Here's how the part is built. I have some questions about the finished solid (model axes, mm). A direction names the side the tool comes from. Coordinates: 2 decimals unless noted, no trailing zeros. Order: outer loops, then holes, each group sorted by start corner. A loop starts at its lowest first (then second) coordinate and runs counter-clockwise, first axis right, second up. Notation, with made-up numbers: (64, 69.5) - (95, 69.5) arc R20 cw to (95, 75.5) - close; hole circle Ø8 at (39.25, 10.25). An arc over 180 degrees is marked (long way). Answer in a Markdown table with one row per item. Add a question column.
Item 1: I want a section at A-A (y = -1.75). Please give me the cut outline in (x, z).
Item 2: I want a section at B-B (x = 15). Please give me the cut outline in (y, z), plus the area to 3 significant figures.
Item 3: If I drill on line 1 along Y through (x, z) = (11.5, 16.5); line 2 along Z through (x, y) = (15, -14.05); line 3 along X through (y, z) = (-7.5, 5.75), over which ranges is the centre line in solid material (lowest first)? Write a range as from..to.
Item 4: I want a section at C-C (z = 11.75). Please give me the cut outline in (x, y).
Item 5: I want a section at D-D (z = 18). Please give me the cut outline in (x, y).
Item 6: On a 3-axis mill with a long thin cutter (end or side, diameter ignored), from which of +Z, -Z, +X, -X, +Y, -Y can I reach the whole of each face in a straight line? I mean faces 4 (the flat face through (2.5, -8, 9)), 5 (the flat face through (2, -7, 15)), 6 (the flat face through (22.652, -13.732, 16.332)). Say none if no direction works.
Item 7: Thinking about a two-plate mould opening in Y: for faces 1 (the flat face through (18, -2.5, 7)), 2 (the flat face through (0, -8, 7)), 3 (the flat face through (14, 0, 6)), which applies, +Y half, -Y half, draft (parallel to the pull), parting line (faces both ways), or undercut?
Item 8: Will these pins go through, and if not, where does the flat tip stop? pin 1 Ø2 at (y, z) = (-14.5, 17) entering from -X; pin 2 Ø5 at (x, y) = (4.5, -4.5) entering from -Z; pin 3 Ø2 at (x, y) = (4, -5.5) entering from +Z; pin 4 Ø4 at (x, y) = (29, -12.5) entering from +Z.
```python
from build123d import *

# Parameters (mm, degrees)
F1_DEPTH = 15
F2_W     = 10
F2_H     = 7.5
F2_H_2   = 12.5
F3_DEPTH = 40
F4_R     = 3.75
F5_DEPTH = 29
F6_W     = 2.5
F6_H     = 10
F7_DEPTH = 12.5


with BuildPart() as f1:
    # F0 (on Front) → F1 (new body)
    with BuildSketch(Plane.XZ):
        Polygon((0, 15), (0, 0), (36.2, 0), (28.829492, 12.766094), (16.3, 20), (7.5, 20), (7.5, 15), align=None)
    extrude(amount=F1_DEPTH)

    # F2 (on face) → F3 (cut)
    with BuildSketch(Plane(origin=(0, 0, 0), x_dir=(0, -1, 0), z_dir=(-1, 0, 0))):
        with Locations((7.5, 18.75)):
            Rectangle(F2_W, F2_H)
        with Locations((7.5, 8.75)):
            Rectangle(F2_W, F2_H_2)
    extrude(amount=-F3_DEPTH, mode=Mode.SUBTRACT)

    # F4 (on face) → F5 (cut)
    with BuildSketch(Plane.XZ.offset(15)):
        with Locations((15, 10)):
            Circle(F4_R)
    extrude(amount=-F5_DEPTH, mode=Mode.SUBTRACT)

    # F6 (on face) → F7 (join)
    with BuildSketch(Plane.XY.offset(2.5)):
        with Locations((1.25, -7.5)):
            Rectangle(F6_W, F6_H)
    extrude(amount=F7_DEPTH)


solid = f1.part
```
Values follow:
| question | item | result |
|---|---|---|
| 1 | outline | (0, 0) - (36.2, 0) - (28.83, 12.77) - (16.3, 20) - (7.5, 20) - (7.5, 15) - (0, 15) - close; hole circle Ø7.5 at (15, 10) |
| 2 | outline | (-15, 0) - (0, 0) - (0, 6.25) - (-2.5, 6.25) - (-2.5, 2.5) - (-12.5, 2.5) - (-12.5, 6.25) - (-15, 6.25) - close; (-15, 13.75) - (-12.5, 13.75) - (-12.5, 20) - (-15, 20) - close; (-2.5, 13.75) - (0, 13.75) - (0, 20) - (-2.5, 20) - close |
| 2 | area | 87.5 mm^2 |
| 3 | line 1 | y = -15..-12.5, -2.5..0 |
| 3 | line 2 | z = 0..6.25, 13.75..20 |
| 3 | line 3 | x = 0..2.5 |
| 4 | outline | (0, -15) - (11.68, -15) - (11.68, -12.5) - (2.5, -12.5) - (2.5, -2.5) - (11.68, -2.5) - (11.68, 0) - (0, 0) - close; (18.32, -15) - (29.42, -15) - (29.42, -12.5) - (18.32, -12.5) - close; (18.32, -2.5) - (29.42, -2.5) - (29.42, 0) - (18.32, 0) - close |
| 5 | outline | (7.5, -15) - (19.76, -15) - (19.76, -12.5) - (7.5, -12.5) - close; (7.5, -2.5) - (19.76, -2.5) - (19.76, 0) - (7.5, 0) - close |
| 6 | face 4 | +Z, +X |
| 6 | face 5 | +Z, -X, +Y, -Y |
| 6 | face 6 | +Z, +X, +Y, -Y |
| 7 | face 1 | undercut |
| 7 | face 2 | draft |
| 7 | face 3 | +Y half |
| 8 | pin 1 | stops at x = 7.5 |
| 8 | pin 2 | stops at z = 0 |
| 8 | pin 3 | stops at z = 2.5 |
| 8 | pin 4 | stops at z = 13.82 |
